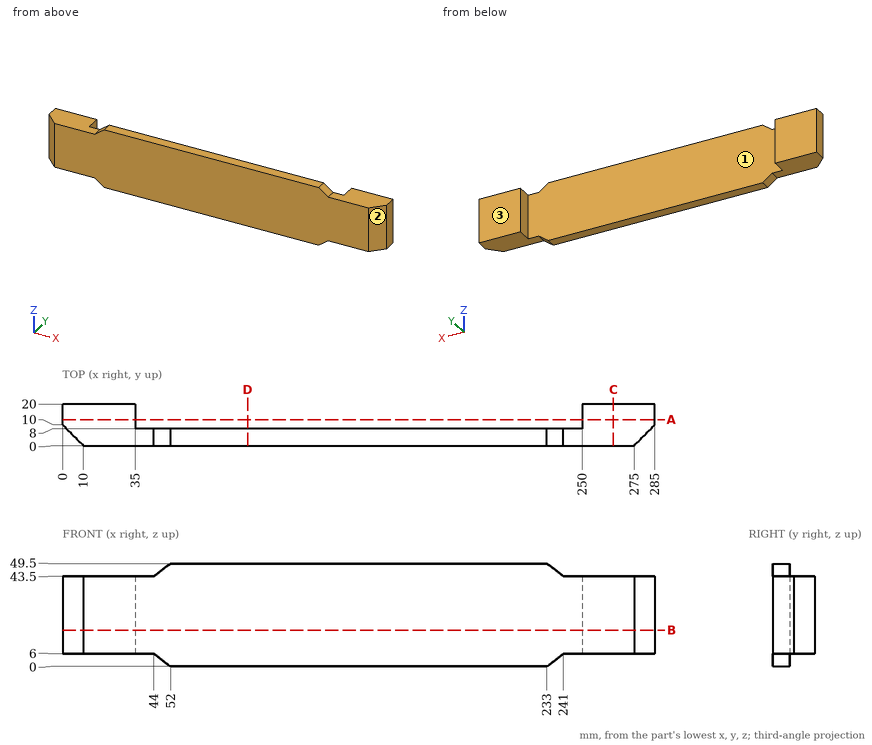
Geometry check sheet. Reference: drawing and pictorial views, mm from the part's lowest x, y, z. Round coordinates to 2 decimals unless told otherwise and drop trailing zeros. Loops run counter-clockwise (first coordinate to the right, second up) from the corner with the lowest first, then second, coordinate; pieces in that order, holes last. Notation, with made-up numbers: (-39.75, 74.25) - (-7.75, 74.25) arc R33 cw to (-7.75, 104.25) - close; hole circle Ø9 at (-16.5, 42.5). An arc over 180 degrees is marked (long way). One line per question, with ' | ' between items. Start each with the question number.
1. Cross-section at A-A on y = 12.5. Record the cut outline in (x, z), then the cut area to 4 significant figures.
2. Cross-section at D-D on x = 89. Record the cut outline in (y, z), then the cut area to 3 significant figures.
3. Scan lines: line 1 (X direction, y = 13.25, z = 37.5); line 2 (Y direction, x = 79, z = 43.5); line 3 (Z direction, x = 35, y = 5.75). Record each from-to range of solid material in increasing order. Write a range as [from, to].
4. Depth check by flat-ended pin: pin 1 (12 mm diameter, centred on x = 217, z = 38.5, fed in from +Y); pin 2 (4 mm diameter, centred on y = 2, z = 18.5, fed in from -X); pin 3 (10 mm diameter, centred on x = 252.5, y = 7, fed in from -Z). Enter the tip coordinate at first touch or a pass-through.
5. Draft check along X on the marked faces 1, 2 and 3. Enter one of: released by +X, released by -X, zero draft, split by the parting line, or undercut.
6. Cross-section at B-B on z = 17.5. Record the cut outline in (x, y), then the cut area to 3 significant figures.
7. Cross-section at C-C on x = 265. Record the cut outline in (y, z), then the cut area to 3 significant figures.
Taken from the geometry:
1) outline: (0, 6) - (35, 6) - (35, 43.5) - (0, 43.5) - close; (250, 6) - (285, 6) - (285, 43.5) - (250, 43.5) - close | area: 2,625 mm²
2) outline: (0, 0) - (8, 0) - (8, 49.5) - (0, 49.5) - close | area: 396 mm²
3) line 1: [0, 35], [250, 285] | line 2: [0, 8] | line 3: [6, 43.5]
4) pin 1: y = 8 | pin 2: x = 6 | pin 3: z = 6
5) face 1: undercut | face 2: released by +X | face 3: zero draft
6) outline: (0, 10) - (10, 0) - (275, 0) - (285, 10) - (285, 20) - (250, 20) - (250, 8) - (35, 8) - (35, 20) - (0, 20) - close | area: 3,020 mm²
7) outline: (0, 6) - (20, 6) - (20, 43.5) - (0, 43.5) - close | area: 750 mm²
